Autodesk Inventor part; units mm, degrees
ref_plane "YZ Plane" through (0, 0, 0) normal (1, 0, 0) x (0, 1, 0)
ref_plane "XZ Plane" through (0, 0, 0) normal (0, 1, 0) x (-1, 0, 0)
ref_plane "XY Plane" through (0, 0, 0) normal (0, 0, 1) x (1, 0, 0)
sketch "Sketch1" plane through (0, 0, 0) normal (1, 0, 0) x (0, 1, 0)
  circle A0 centre (0, 0) radius 3.175
  dimension "d0" = 6.35
extrude "Extrusion1" add sketch "Sketch1" along normal blind 50.8
sketch "Sketch2" plane through (0, 0, 0) normal (0, 1, 0) x (-1, 0, 0)
  circle A0 centre (-5.08, 0) radius 1.27
  line L0 (0, 3.175) -> (0, -3.175)
  point P0 (0, 0)
  dimension "d3" = 2.54
  dimension "d4" = 5.08
extrude "Extrusion2" cut sketch "Sketch2" along normal mid plane 50.8
sketch "Sketch3" plane through (0, 0, 0) normal (0, 1, 0) x (-1, 0, 0)
  circle A0 centre (-45.72, 0) radius 1.27
  line L0 (-50.8, 3.175) -> (-50.8, -3.175)
  point P0 (0, 0)
  dimension "d7" = 2.54
  dimension "d8" = 5.08
extrude "Extrusion3" cut sketch "Sketch3" along normal mid plane 50.8
properties part number "TIE ROD"
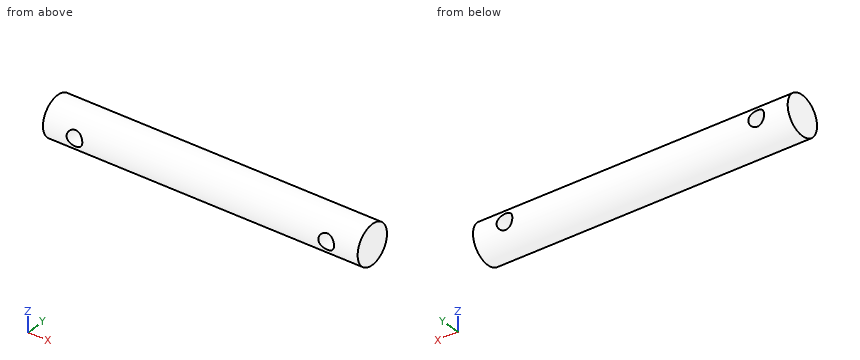
Design review of the part built by this model. Coordinates are the model's own, in mm. Give positions to 0.01 mm unless a question says otherwise; leave off trailing zeros. Order: outer loops, then holes, each group sorted by start corner. A loop starts at its lowest first (then second) coordinate and runs counter-clockwise, first axis right, second up. Notation, with made-up numbers: (-15.5, 79) - (41.5, 79) arc R9 cw to (41.5, 91) - close; hole circle Ø8 at (50, 51). An arc over 180 degrees is marked (long way). Use CSV: the item, a comma, the result in double quotes. Start each with the question number.
Q1. For P1, Ø1.5, axis at x = 14.5, y = -1, coming from the -Z side; P2, Ø1, axis at x = 45, z = 1.5, coming from the -Y side; P3, Ø1, axis at x = 35.5, z = 2.5, coming from the +Y side, all flat-tipped, find the tip position at first contact; note any pin that passes through.
Q2. For line 1 (X direction, y = 1.75, z = 0); line 2 (X direction, y = 2.25, z = -0.5); line 3 (Z direction, x = 45.72, y = 0) (3 decimals), list the stretches that pass through material, from the lowest coordinate up.
Q3. Take a section at A-A (z = 0). State the section outline as (x, y) points (3 decimals), and give its area (3 significant figures).
Q4. Take a section at D-D (x = 4.5). State the section outline as (y, z) points (3 decimals).
Q5. Take a section at B-B (y = 0). State the section outline as (x, z) points (3 decimals).
Q6. Take a section at C-C (x = 10). State the section outline as (y, z) points (3 decimals).
Calculated:
1,P1,"stops at z = -3.17"
1,P2,"stops at y = -3.01"
1,P3,"stops at y = 2.47"
2,line 1,"x = 0 to 3.81, 6.35 to 44.45, 46.99 to 50.8"
2,line 2,"x = 0 to 3.91, 6.25 to 44.55, 46.89 to 50.8"
2,line 3,"z = -3.175 to -1.27, 1.27 to 3.175"
3,outline,"(0, -3.175) - (3.81, -3.175) - (3.81, 3.175) - (0, 3.175) - close; (6.35, -3.175) - (44.45, -3.175) - (44.45, 3.175) - (6.35, 3.175) - close; (46.99, -3.175) - (50.8, -3.175) - (50.8, 3.175) - (46.99, 3.175) - close"
3,area,"290 mm²"
4,outline,"(-2.967, -1.13) arc R3.175 ccw to (2.967, -1.13) - close; (-2.967, 1.13) - (2.967, 1.13) arc R3.175 ccw to start"
5,outline,"(0, -3.175) - (50.8, -3.175) - (50.8, 3.175) - (0, 3.175) - close; hole circle Ø2.54 at (5.08, 0); hole circle Ø2.54 at (45.72, 0)"
6,outline,"circle Ø6.35 at (0, 0)"
